The listing builds one solid part. Answer for the finished solid, in the listing's coordinates (mm). Face numbers are marked on the shaded views. A direction names the side the tool comes from. Coordinates: 2 decimals unless noted, no trailing zeros. Order: outer loops, then holes, each group sorted by start corner. A loop starts at its lowest first (then second) coordinate and runs counter-clockwise, first axis right, second up. Notation, with made-up numbers: (40.25, 9) -> (69.25, 9) arc R20 ccw to (69.25, 40) -> close; hole circle Ø7 at (57.5, 58). An arc over 180 degrees is marked (long way). Return JSON: item names as keys, results as strings.
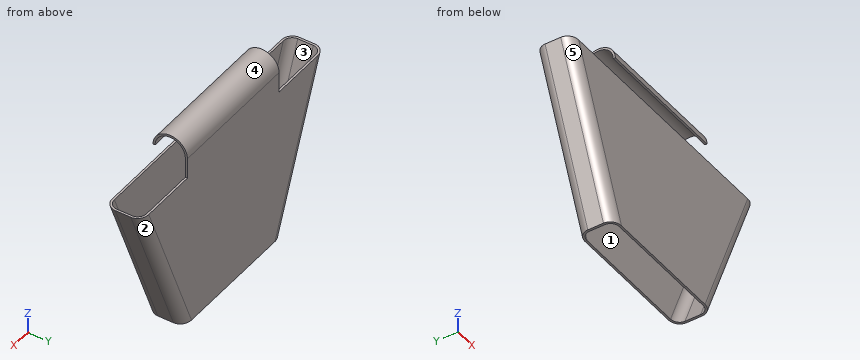
```python
from build123d import *

# Parameters (mm, degrees)
F1_DEPTH = 4.445
F2_R     = 2.54
F3_T     = -0.508
F6_DEPTH = 16.51


with BuildPart() as f1:
    # F0 (on Front) → F1 (new body, symmetric)
    with BuildSketch(Plane.XZ):
        Polygon((17.78, -38.1), (33.173399, 0), (-33.173399, 0), (-17.78, -38.1), align=None)
    extrude(amount=F1_DEPTH, both=True)

    # F2
    f2_edges = [f1.edges().sort_by_distance(p)[0] for p in [
        (25.4767, 4.445, -19.05),
        (25.4767, -4.445, -19.05),
        (-25.4767, 4.445, -19.05),
        (-25.4767, -4.445, -19.05),
    ]]
    fillet(f2_edges, radius=F2_R)

    # F3
    f3_openings = [f1.faces().sort_by_distance(p)[0] for p in [
        (0, 0, 0),
        (0, 0, -38.1),
    ]]
    offset(amount=F3_T, openings=f3_openings)

    # F5 (on Right) → F6 (join, symmetric)
    with BuildSketch(Plane.YZ):
        with BuildLine():
            Line((3.937, 0), (4.445, 0))
            Line((4.445, 0), (4.445, 5.08))
            ThreePointArc((4.445, 5.08), (0.254, 9.271), (-3.937, 5.08))
            Line((-3.937, 5.08), (-3.429, 5.08))
            ThreePointArc((-3.429, 5.08), (0.254, 8.763), (3.937, 5.08))
            Line((3.937, 5.08), (3.937, 0))
        make_face()
    extrude(amount=F6_DEPTH, both=True)


solid = f1.part
```
Item 1: Find the intervals of material crossed by probe 1 along Y at (x, z) = (2, -28) (3 decimals); probe 2 along Z at (x, y) = (-14.5, 0.5); probe 3 along X at (y, z) = (3.75, -16), in increasing order.
Answer list:
{"probe 1": "-4.445 to -3.937, 3.937 to 4.445", "probe 2": "8.75 to 9.26", "probe 3": "-25.85 to -24.89, 24.89 to 25.85"}
Item 2: Determine the mould class of the marked faces 3, 4 and 5 for opening direction X: pulls with the +X half, pulls with the -X half, needs draft (parallel to the pull), parting line crosses it, or undercut.
Answer list:
{"face 3": "undercut", "face 4": "needs draft", "face 5": "pulls with the -X half"}
Item 3: Flat-ended cylindrical pins translate along their axes: pin 1 (4 mm diameter, centred on x = 22, y = -1, fed in from +Z); pin 2 (2 mm diameter, centred on y = -2, z = -19.5, fed in from +X); pin 3 (3 mm diameter, centred on y = -2.5, z = -9.5, fed in from -X). Find the tip coordinate at first contact, or state that the pin passes through.
Answer list:
{"pin 1": "z = -21.35", "pin 2": "x = 25.7", "pin 3": "x = -29.91"}
Item 4: Which of the six approach directions +Z, -Z, +X, -X, +Y, -Y give full straight-line access (tool end or side, diameter ignored) to the marked faces 1 and 2?
Answer list:
{"face 1": "none", "face 2": "-Z, +X, +Y"}
Item 5: The part is cut by section B-B on y = 0.5. Determine the outline of the cut face in (x, z).
Answer list:
{"outline": "(-33.17, 0) -> (-17.78, -38.1) -> (-17.23, -38.1) -> (-32.63, 0) -> close; (-16.51, 8.75) -> (16.51, 8.75) -> (16.51, 9.26) -> (-16.51, 9.26) -> close; (17.23, -38.1) -> (17.78, -38.1) -> (33.17, 0) -> (32.63, 0) -> close"}
Item 6: The part is cut by section A-A on x = 14. Determine the outline of the cut face in (y, z) (3 decimals), plus the area to 3 significant figures.
Answer list:
{"outline": "(-4.445, -38.1) -> (-3.937, -38.1) -> (-3.937, 0) -> (-4.445, 0) -> close; (-3.937, 5.08) -> (-3.429, 5.08) arc R3.683 cw to (3.937, 5.08) -> (3.937, -38.1) -> (4.445, -38.1) -> (4.445, 5.08) arc R4.191 ccw to start", "area": "47.6 mm2"}
